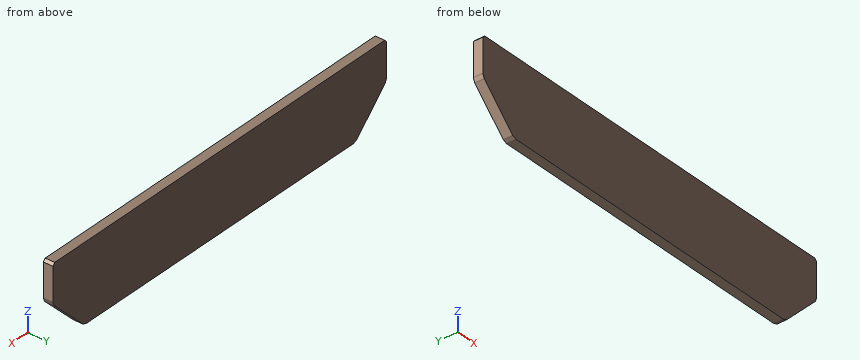
```python
from build123d import *

# Parameters (mm, degrees)
SKETCH_W        = 770
SKETCH_H        = 144.4
PAD_DEPTH       = 9
CHAMFER_SIZE    = 72.2
CHAMFER001_SIZE = 4.5


with BuildPart() as part:
    # Sketch → Pad (new body, symmetric)
    with BuildSketch(Plane.XZ):
        with Locations((385, 687.8)):
            Rectangle(SKETCH_W, SKETCH_H)
    extrude(amount=PAD_DEPTH, both=True)

    # Chamfer
    chamfer_edges = [part.edges().sort_by_distance(p)[0] for p in [
        (770, 0, 615.6),
        (0, 0, 615.6),
    ]]
    chamfer(chamfer_edges, length=CHAMFER_SIZE)

    # Chamfer001
    chamfer001_edges = [part.edges().sort_by_distance(p)[0] for p in [
        (0, 0, 687.8),
        (0, 0, 760),
        (72.2, 0, 615.6),
        (697.8, 0, 615.6),
        (770, 0, 687.8),
        (770, 0, 760),
    ]]
    chamfer(chamfer001_edges, length=CHAMFER001_SIZE)


solid = part.part
```
Here's how the part is built. I have some questions about the finished solid (model axes, mm). Coordinates: 2 decimals unless noted, no trailing zeros. Loops run counter-clockwise (first coordinate to the right, second up) from the corner with the lowest first, then second, coordinate; pieces in that order, holes last. Notation, with made-up numbers: (52, -19.5) - (59, -19.5) arc R19 cw to (59, 3.5) - close; hole circle Ø9 at (52, 33). An arc over 180 degrees is marked (long way). Answer as CSV lines item,"result".
Q1. If we section it at C-C, the plane x = 718: Write out the boundary of the cut face in (y, z), and give its area (3 significant figures).
Response:
outline,"(-9, 635.8) - (9, 635.8) - (9, 760) - (-9, 760) - close"
area,"2,240 mm2"
Q2. If we section it at A-A, the plane y = 2.75: Write out the boundary of the cut face in (x, z), and give its area (3 significant figures).
Response:
outline,"(0, 692.3) - (3.18, 684.62) - (69.02, 618.78) - (76.7, 615.6) - (693.3, 615.6) - (700.98, 618.78) - (766.82, 684.62) - (770, 692.3) - (770, 755.5) - (765.5, 760) - (4.5, 760) - (0, 755.5) - close"
area,"106,000 mm2"
Q3. If we section it at B-B, the plane z = 655: Write out the boundary of the cut face in (x, y), and give its area (3 significant figures).
Response:
outline,"(32.8, -9) - (737.2, -9) - (737.2, 9) - (32.8, 9) - close"
area,"12,700 mm2"
Q4. If I drill on L1, parallel to X at y = -1.25, z = 635.5; L2, parallel to X at y = -2.25, z = 667; L3, parallel to Z at x = 696, y = 1.25, over which ranges is the centre line in solid material (lowest first)? Write a range as [from, to].
Response:
L1,"[52.3, 717.7]"
L2,"[20.8, 749.2]"
L3,"[616.72, 760]"
Q5. For pin 1 (5 mm diameter, centred on y = 5.5, z = 667, fed in from -X), with a flat end and sliding along its axis, tell me the tip position at first contact or that it passes through.
Response:
pin 1,"x = 18.3"
